```python
from build123d import *

# Parameters (mm, degrees)
SKETCH2_R               = 32.5
BOSS_EXTRUDE1_DEPTH     = 160
CUT_EXTRUDE2_DEPTH      = 50
CUT_EXTRUDE2_DEPTH_BACK = 50
SKETCH4_W               = 130
SKETCH4_H               = 15
CUT_EXTRUDE3_DEPTH      = 50
CUT_EXTRUDE3_DEPTH_BACK = 50
SKETCH5_W               = 130
SKETCH5_H               = 15
FILLET2_START           = 11.9999999
FILLET2_DEPTH           = 136.0000002
SKETCH6_R               = 29
CUT_EXTRUDE4_DEPTH      = 160
FILLET3_R               = 8


with BuildPart() as part:
    # Sketch2 → Boss-Extrude1 (new body)
    with BuildSketch(Plane(origin=(0, 0, 0), x_dir=(0, 0, -1), z_dir=(1, 0, 0))):
        Circle(SKETCH2_R)
    extrude(amount=BOSS_EXTRUDE1_DEPTH)

    # Sketch4 → Cut-Extrude2 (cut, two sides: drawn at the far end of the back side and taken through both)
    with BuildSketch(Plane.XY.offset(-CUT_EXTRUDE2_DEPTH_BACK)):
        with Locations((80, 0)):
            Rectangle(SKETCH4_W, SKETCH4_H)
    extrude(amount=CUT_EXTRUDE2_DEPTH + CUT_EXTRUDE2_DEPTH_BACK, mode=Mode.SUBTRACT)

    # Sketch5 → Cut-Extrude3 (cut, two sides: drawn at the far end of the back side and taken through both)
    with BuildSketch(Plane(origin=(0, 0, 0), x_dir=(1, 0, 0), z_dir=(0, 1, 0)).offset(-CUT_EXTRUDE3_DEPTH_BACK)):
        with Locations((80, 0)):
            Rectangle(SKETCH5_W, SKETCH5_H)
    extrude(amount=CUT_EXTRUDE3_DEPTH + CUT_EXTRUDE3_DEPTH_BACK, mode=Mode.SUBTRACT)

    # Fillet2: read off the stored shape, not the designer's step
    # Fillet2 outline → Fillet2 (cut)
    with BuildSketch(Plane.YZ.offset(FILLET2_START)):
        with BuildLine():
            ThreePointArc((-30.371632844, 11.56779661), (-32.5, 0), (-30.371632844, -11.56779661))
            ThreePointArc((-30.371632844, -11.56779661), (-30.038258413, -8.79755908), (-27.568097504, -7.5))
            Line((-27.568097504, -7.5), (-7.5, -7.5))
            Line((-7.5, -7.5), (-7.5, -27.568097504))
            ThreePointArc((-7.5, -27.568097504), (-8.79755908, -30.038258413), (-11.56779661, -30.371632844))
            ThreePointArc((-11.56779661, -30.371632844), (0, -32.5), (11.56779661, -30.371632844))
            ThreePointArc((11.56779661, -30.371632844), (8.79755908, -30.038258413), (7.5, -27.568097504))
            Line((7.5, -27.568097504), (7.5, -7.5))
            Line((7.5, -7.5), (27.568097504, -7.5))
            ThreePointArc((27.568097504, -7.5), (30.038258413, -8.79755908), (30.371632844, -11.56779661))
            ThreePointArc((30.371632844, -11.56779661), (32.5, 0), (30.371632844, 11.56779661))
            ThreePointArc((30.371632844, 11.56779661), (30.038258413, 8.79755908), (27.568097504, 7.5))
            Line((27.568097504, 7.5), (7.5, 7.5))
            Line((7.5, 7.5), (7.5, 27.568097504))
            ThreePointArc((7.5, 27.568097504), (8.79755908, 30.038258413), (11.56779661, 30.371632844))
            ThreePointArc((11.56779661, 30.371632844), (0, 32.5), (-11.56779661, 30.371632844))
            ThreePointArc((-11.56779661, 30.371632844), (-8.79755908, 30.038258413), (-7.5, 27.568097504))
            Line((-7.5, 27.568097504), (-7.5, 7.5))
            Line((-7.5, 7.5), (-27.568097504, 7.5))
            ThreePointArc((-27.568097504, 7.5), (-30.038258413, 8.79755908), (-30.371632844, 11.56779661))
        make_face()
    extrude(amount=FILLET2_DEPTH, mode=Mode.SUBTRACT)

    # Fillet2 2 outline → Fillet2 2 (revolve)
    with BuildSketch(Plane.YX):
        with BuildLine():
            Line((0, 148.0000001), (0, 145))
            Line((0, 145), (29.5, 145))
            ThreePointArc((29.5, 145), (31.621320344, 145.878679656), (32.5, 148))
            Line((32.5, 148), (0, 148.0000001))
        make_face()
        with BuildLine():
            Line((29.5, 15), (0, 15))
            Line((0, 15), (0, 11.9999999))
            Line((0, 11.9999999), (32.5, 12))
            ThreePointArc((32.5, 12), (31.621320344, 14.121320344), (29.5, 15))
        make_face()
    revolve(axis=Axis((0, 0, 0), (1, 0, 0)))

    # Sketch6 → Cut-Extrude4 (cut)
    with BuildSketch(Plane(origin=(170, 0, 0), x_dir=(0, 0, -1), z_dir=(1, 0, 0))):
        Circle(SKETCH6_R)
    extrude(amount=-CUT_EXTRUDE4_DEPTH, mode=Mode.SUBTRACT)

    # Fillet3
    # the kernel refuses this fillet: 8 mm, written as the material it takes off along each edge
    with BuildSketch(Plane(origin=(0, 0, 0), x_dir=(0, 0, -1), z_dir=(0, -1, 0))) as fillet3_piece_1:
        with BuildLine():
            CenterArc((32.5 - FILLET3_R, FILLET3_R), FILLET3_R, 270, 90)
            Line((32.5 - FILLET3_R, 0), (32.5 - FILLET3_R, -FILLET3_R * 0.02))
            Line((32.5 - FILLET3_R, -FILLET3_R * 0.02), (32.5 + FILLET3_R * 0.02, -FILLET3_R * 0.02))
            Line((32.5 + FILLET3_R * 0.02, -FILLET3_R * 0.02), (32.5 + FILLET3_R * 0.02, FILLET3_R))
            Line((32.5 + FILLET3_R * 0.02, FILLET3_R), (32.5, FILLET3_R))
        make_face()
    revolve(axis=Axis((0, 0, 0), (1, 0, 0)), mode=Mode.SUBTRACT)
    with BuildSketch(Plane(origin=(160, 0, 0), x_dir=(0, 0, -1), z_dir=(0, -1, 0))) as fillet3_piece_2:
        with BuildLine():
            CenterArc((24.5, -6.614378278), FILLET3_R, 0, 55.771133672)
            Line((29, 0), (29.09, 0.132287566))
            ThreePointArc((29.09, 0.132287566), (30.75, 0.16), (32.5, 0.16))
            Line((32.5, 0.16), (32.66, 0))
            Line((32.66, 0), (32.66, -6.614378278))
            Line((32.66, -6.614378278), (32.5, -6.614378278))
        make_face()
    revolve(axis=Axis((160, 0, 0), (1, 0, 0)), mode=Mode.SUBTRACT)


solid = part.part
```
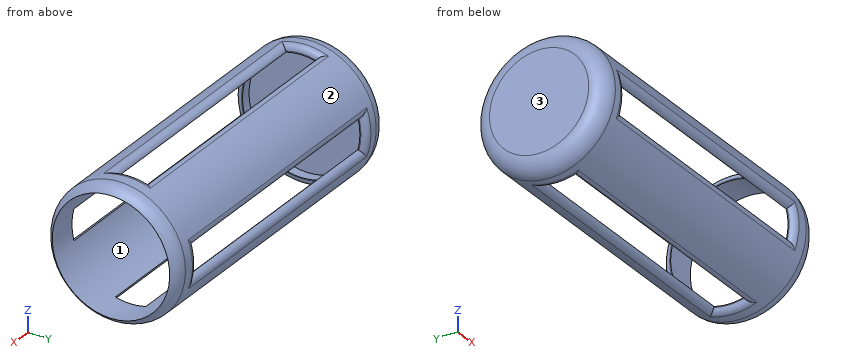
The model under review builds one solid part; all positions refer to its coordinate system, in mm. Face numbers are marked on the shaded views. Coordinates: 2 decimals unless noted, no trailing zeros. Write each loop counter-clockwise with the first axis right and the second up, starting at its lowest first coordinate (ties: lowest second). Pieces come first, ordered by that corner, then holes. Notation, with made-up numbers: (12.5, -17) - (28.5, -17) arc R16 cw to (28.5, 0) - close; hole circle Ø10 at (12.25, 7.5). An arc over 180 degrees is marked (long way). Answer in a Markdown table with one row per item. Add a question column.
Q1. To check wall thickness, follow line 1 along X through (y, z) = (-3, 4); line 2 along Y through (x, z) = (143, -14); line 3 along Z through (x, y) = (80, 9). State the ranges of each line that lie inside material, in increasing order. Write a range as from..to.
Q2. Consider section A-A on z = 0. Give the boundary of the cut face in (x, y).
Q3. Draft analysis for pull direction Z (two halves, no side actions). For the marked faces 1, 2 and 3, state which applies: +Z half, -Z half, draft (parallel to the pull), parting line (faces both ways), or undercut.
Q4. Clearance check with flat-ended pins moving along their axes: pin 1 (1.6 mm diameter, centred on y = 2, z = 29, fed in from -X); pin 2 (3 mm diameter, centred on x = 44, z = -17, fed in from -Y); pin 3 (5 mm diameter, centred on x = 121.5, y = -8, fed in from -Z); pin 4 (1.2 mm diameter, centred on y = -1.5, z = -29, fed in from +X). State where each tip first meets the part, or that it passes through.
Q5. Consider section C-C on x = 129. Give the boundary of the cut face in (y, z), then the cut area to 3 significant figures.
Answers below:
| question | item | result |
|---|---|---|
| 1 | line 1 | 0..10 |
| 1 | line 2 | -29.33..-25.4, 25.4..29.33 |
| 1 | line 3 | -30.17..-27.57, 27.57..30.17 |
| 2 | outline | (0, -24.5) arc R8 ccw to (8, -32.5) - (12, -32.5) arc R3 ccw to (15, -29.5) - (15, -29) - (10, -29) - (10, 29) - (15, 29) - (15, 29.5) arc R3 ccw to (12, 32.5) - (8, 32.5) arc R8 ccw to (0, 24.5) - close; (145, -29.5) arc R3 ccw to (148, -32.5) - (153.39, -32.5) arc R8 ccw to (160, -29) - (145, -29) - close; (145, 29) - (160, 29) arc R8 ccw to (153.39, 32.5) - (148, 32.5) arc R3 ccw to (145, 29.5) - close |
| 3 | face 1 | undercut |
| 3 | face 2 | parting line |
| 3 | face 3 | draft |
| 4 | pin 1 | x = 0.94 |
| 4 | pin 2 | y = -28.57 |
| 4 | pin 3 | z = -30.57 |
| 4 | pin 4 | x = 160 |
| 5 | outline | (-30.37, -11.57) arc R32.5 ccw to (-11.57, -30.37) arc R3 ccw to (-7.53, -28) arc R29 cw to (-28, -7.53) arc R3 ccw to start; (-30.37, 11.57) arc R3 ccw to (-28, 7.53) arc R29 cw to (-7.53, 28) arc R3 ccw to (-11.57, 30.37) arc R32.5 ccw to start; (7.53, -28) arc R3 ccw to (11.57, -30.37) arc R32.5 ccw to (30.37, -11.57) arc R3 ccw to (28, -7.53) arc R29 cw to start; (7.53, 28) arc R29 cw to (28, 7.53) arc R3 ccw to (30.37, 11.57) arc R32.5 ccw to (11.57, 30.37) arc R3 ccw to start |
| 5 | area | 433 mm² |
